Source: CAD feature listing. Evaluate the final solid. Frame: model axes, mm. A direction names the side the tool comes from. Give positions to 0.01 mm unless a question says otherwise; leave off trailing zeros. Order: outer loops, then holes, each group sorted by start corner. A loop starts at its lowest first (then second) coordinate and runs counter-clockwise, first axis right, second up. Notation, with made-up numbers: M -16.75,-4 L 5.25,-4 A24 ccw 5.25,19 Z; hole C 56,55.5 d7. An arc over 180 degrees is marked long. Answer as a JSON object with one key per item and string values. Group by question number.
1. Pin query (flat end, axial travel): P1, Ø9, axis at x = 12.7, y = -11.11, coming from the +Z side; P2, Ø5, axis at x = 17.5, y = -88.5, coming from the -Z side. Return the tip coordinate at first contact, or that it passes through.
2. Section query B-B (y = -59). Output: boundary loops of the cut face in (x, z) (1 decimal).
3. Section query C-C (z = 3.75). Count the separate pieces of the cut face and the enclosed holes in it, plus the area to 3 significant figures.
4. Pull-direction query (Y, two-part tool) for faces 4 (the flat face through (19, -20.638, 5)), 5 (the cylindrical face through (24.45, -94.34, 8.61)), 6 (the flat face through (15, -11, 12.7)), 7 (the flat face through (13, 0, 9)); classes: +Y half, -Y half, draft (parallel to the pull), parting line (faces both ways), or undercut.
5. Material intervals for L1, parallel to X at y = -89, z = 5.5; L2, parallel to Y at x = 12.7, z = 14.75 (3 decimals); L3, parallel to Y at x = 12.7, z = 6.25 (3 decimals), sorted ascending. Write a range as [from, to].
6. Set-up query: faces 1 (the cylindrical face through (8.29, -14.49, 15.11)), 2 (the flat face through (13, -73.025, 9)), 3 (the flat face through (11.906, -5, 5)). Return all of +Z, -Z, +X, -X, +Y, -Y with unobstructed straight access to the full face (end or side cutting, diameter ignored); none if empty.
from build123d import *

# Parameters (mm, degrees)
F1_DEPTH = 17.4625
F3_R     = 1.984375
F4_DEPTH = 17.4635
F5_DEPTH = 3.175
F6_R     = 1.984375
F7_DEPTH = 11.1125
F8_R     = 5.55625
F8_R_2   = 1.984375
F9_DEPTH = 4.7625


with BuildPart() as f1:
    # F0 (on Top) → F1 (new body)
    with BuildSketch(Plane.XY):
        with BuildLine():
            Line((22.225, 0), (3.175, 0))
            ThreePointArc((3.175, 0), (0.9299359697, -0.9299359697), (0, -3.175))
            Line((0, -3.175), (0, -92.075))
            ThreePointArc((0, -92.075), (0.9299359697, -94.3200640303), (3.175, -95.25))
            Line((3.175, -95.25), (22.225, -95.25))
            ThreePointArc((22.225, -95.25), (24.4700640303, -94.3200640303), (25.4, -92.075))
            Line((25.4, -92.075), (25.4, -3.175))
            ThreePointArc((25.4, -3.175), (24.4700640303, -0.9299359697), (22.225, 0))
        make_face()
        Polygon((3.175, -22.225), (12.7, -22.225), (22.225, -22.225), (22.225, -47.625), (22.225, -73.025), (12.7, -73.025), (3.175, -73.025), (3.175, -47.625), align=None, mode=Mode.SUBTRACT)
    extrude(amount=F1_DEPTH)

    # F3 (on face) → F4 (cut, through all)
    with BuildSketch(Plane(origin=(0, 0, 0), x_dir=(1, 0, 0), z_dir=(0, 0, -1))):
        with Locations((12.7, 11.1125)):
            Circle(F3_R)
        with Locations((12.7, 84.1375)):
            Circle(F3_R)
    extrude(amount=-F4_DEPTH, mode=Mode.SUBTRACT)

    # F0 (on Top) → F5 (cut)
    with BuildSketch(Plane.XY):
        Polygon((22.225, -22.225), (12.7, -22.225), (3.175, -22.225), (3.175, -47.625), (3.175, -73.025), (12.7, -73.025), (22.225, -73.025), (22.225, -47.625), align=None)
    extrude(amount=F5_DEPTH, mode=Mode.SUBTRACT)

    # F6 (on face) → F7 (cut)
    with BuildSketch(Plane(origin=(0, 0, 0), x_dir=(1, 0, 0), z_dir=(0, 0, -1))):
        with BuildLine():
            ThreePointArc((11.90625, 80.6549360088), (9.128125, 84.1375), (11.90625, 87.6200639912))
            Line((11.90625, 87.6200639912), (11.90625, 93.6625))
            Line((11.90625, 93.6625), (3.175, 93.6625))
            ThreePointArc((3.175, 93.6625), (2.0524679849, 93.1975320151), (1.5875, 92.075))
            Line((1.5875, 92.075), (1.5875, 74.6125))
            Line((1.5875, 74.6125), (11.90625, 74.6125))
            Line((11.90625, 74.6125), (11.90625, 80.6549360088))
        make_face()
        with BuildLine():
            Line((22.225, 93.6625), (13.49375, 93.6625))
            Line((13.49375, 93.6625), (13.49375, 87.6200639912))
            ThreePointArc((13.49375, 87.6200639912), (16.271875, 84.1375), (13.49375, 80.6549360088))
            Line((13.49375, 80.6549360088), (13.49375, 74.6125))
            Line((13.49375, 74.6125), (23.8125, 74.6125))
            Line((23.8125, 74.6125), (23.8125, 92.075))
            ThreePointArc((23.8125, 92.075), (23.3475320151, 93.1975320151), (22.225, 93.6625))
        make_face()
        with BuildLine():
            Line((11.90625, 20.6375), (1.5875, 20.6375))
            Line((1.5875, 20.6375), (1.5875, 3.175))
            ThreePointArc((1.5875, 3.175), (2.0524679849, 2.0524679849), (3.175, 1.5875))
            Line((3.175, 1.5875), (11.90625, 1.5875))
            Line((11.90625, 1.5875), (11.90625, 7.6299360088))
            ThreePointArc((11.90625, 7.6299360088), (9.128125, 11.1125), (11.90625, 14.5950639912))
            Line((11.90625, 14.5950639912), (11.90625, 20.6375))
        make_face()
        with BuildLine():
            Line((23.8125, 3.175), (23.8125, 20.6375))
            Line((23.8125, 20.6375), (13.49375, 20.6375))
            Line((13.49375, 20.6375), (13.49375, 14.5950639912))
            ThreePointArc((13.49375, 14.5950639912), (16.271875, 11.1125), (13.49375, 7.6299360088))
            Line((13.49375, 7.6299360088), (13.49375, 1.5875))
            Line((13.49375, 1.5875), (22.225, 1.5875))
            ThreePointArc((22.225, 1.5875), (23.3475320151, 2.0524679849), (23.8125, 3.175))
        make_face()
        with Locations((12.7, 11.1125)):
            Circle(F6_R)
    extrude(amount=-F7_DEPTH, mode=Mode.SUBTRACT)

    # F8 (on face) → F9 (cut)
    with BuildSketch(Plane.XY.offset(17.4625)):
        with Locations((12.7, -84.1375)):
            Circle(F8_R)
        with Locations((12.7, -84.1375)):
            Circle(F8_R_2, mode=Mode.SUBTRACT)
        with Locations((12.7, -11.1125)):
            Circle(F8_R)
        with Locations((12.7, -11.1125)):
            Circle(F8_R_2, mode=Mode.SUBTRACT)
        with Locations((12.7, -11.1125)):
            Circle(F8_R_2)
    extrude(amount=-F9_DEPTH, mode=Mode.SUBTRACT)


solid = f1.part
Answer sheet:
{
 "1": {"P1": "z = 12.7", "P2": "z = 11.11"},
 "2": {"outline": "M 0,0 L 3.2,0 L 3.2,17.5 L 0,17.5 Z; M 22.2,0 L 25.4,0 L 25.4,17.5 L 22.2,17.5 Z"},
 "3": {"separate pieces": "1", "enclosed holes": "7", "area": "692 mm^2"},
 "4": {"face 4": "undercut", "face 5": "-Y half", "face 6": "undercut", "face 7": "+Y half"},
 "5": {"L1": "[0, 1.59], [11.91, 13.49], [23.81, 25.4]", "L2": "[-95.25, -89.694], [-78.581, -73.025], [-22.225, -16.669], [-5.556, 0]", "L3": "[-95.25, -86.122], [-82.153, -73.025], [-22.225, -13.097], [-9.128, 0]"},
 "6": {"face 1": "+Z", "face 2": "+Z, -Z", "face 3": "-Z"}
}
